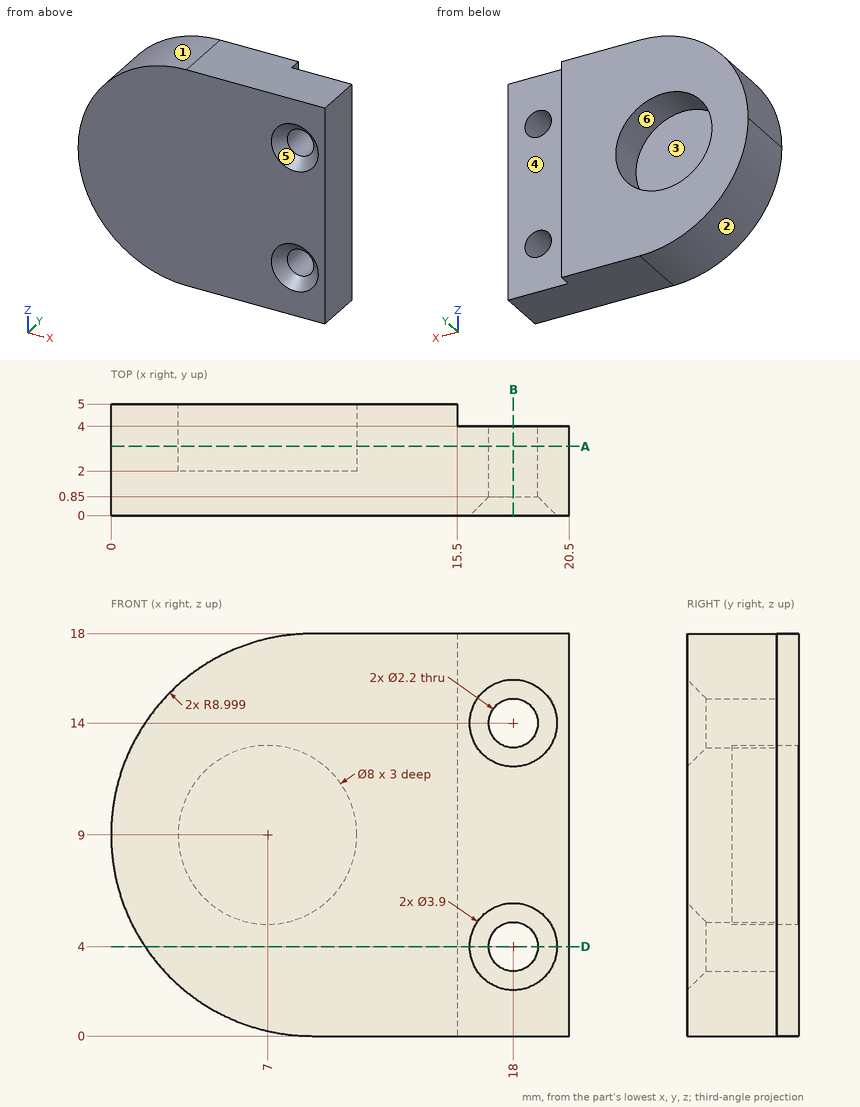
The drawing under review shows one solid part. Ordinate dimensions are in mm from its lowest x, y, z. A direction names the side the tool comes from. Coordinates: 2 decimals unless noted, no trailing zeros. Loops run counter-clockwise (first coordinate to the right, second up) from the corner with the lowest first, then second, coordinate; pieces in that order, holes last. Notation, with made-up numbers: (4, -23.5) - (49, -23.5) arc R16 cw to (49, -14.5) - close; hole circle Ø5 at (83, -6). An arc over 180 degrees is marked (long way). Use CSV: the item, a comma, the result in double quotes. Start each with the question number.
1. Clearance check with flat-ended pins moving along their axes: pin 1 (1.5 mm diameter, centred on y = 3, z = 10.5, fed in from -X); pin 2 (0.5 mm diameter, centred on y = 4.5, z = 7, fed in from +X); pin 3 (5.5 mm diameter, centred on x = 18.5, z = 9.5, fed in from +Y). State where each tip first meets the part, or that it passes through.
2. Add section D-D on z = 4. Give the boundary of the cut face in (x, y).
3. Add section A-A on y = 3.1. Count the separate pieces of the cut face and the enclosed holes in it, plus the area to 3 significant figures.
4. Add section B-B on x = 18. Give the boundary of the cut face in (y, z).
5. Mouldability with a two-part tool opening along Z and no side actions: class the marked faces 1, 2 and 3 as released by +Z, released by -Z, zero draft, split by the parting line, or undercut.
6. For the marked faces 4, 5 and 6, list the 3-axis set-ups (+Z, -Z, +X, -X, +Y, -Y) from which the entire face can be reached by the end or side of a thin tool; tool diameter is ignored.
7. To check wall thickness, follow probe 1 along Z at (x, y) = (18, 2.15); probe 2 along Y at (x, z) = (7.75, 10); probe 3 along X at (y, z) = (3.2, 7) (1 decimal). State the ranges of each line that lie inside material, in increasing order.
Resolved:
1,pin 1,"x = 0.03"
1,pin 2,"x = 15.5"
1,pin 3,"y = 4"
2,outline,"(1.52, 0) - (16.05, 0) - (16.9, 0.85) - (16.9, 4) - (15.5, 4) - (15.5, 5) - (1.52, 5) - close; (19.1, 0.85) - (19.95, 0) - (20.5, 0) - (20.5, 4) - (19.1, 4) - close"
3,separate pieces,"1"
3,enclosed holes,"3"
3,area,"276 mm2"
4,outline,"(0, 0) - (4, 0) - (4, 2.9) - (0.85, 2.9) - (0, 2.05) - close; (0, 5.95) - (0.85, 5.1) - (4, 5.1) - (4, 12.9) - (0.85, 12.9) - (0, 12.05) - close; (0, 15.95) - (0.85, 15.1) - (4, 15.1) - (4, 18) - (0, 18) - close"
5,face 1,"released by +Z"
5,face 2,"released by -Z"
5,face 3,"undercut"
6,face 4,"+Z, -Z, +X, +Y"
6,face 5,"-Y"
6,face 6,"+Y"
7,probe 1,"0 to 2.9, 5.1 to 12.9, 15.1 to 18"
7,probe 2,"0 to 2"
7,probe 3,"0.2 to 3.5, 10.5 to 20.5"
